The listing builds one solid part. Answer for the finished solid, in the listing's coordinates (mm). A direction names the side the tool comes from. Give positions to 0.01 mm unless a question says otherwise; leave off trailing zeros. Loops run counter-clockwise (first coordinate to the right, second up) from the corner with the lowest first, then second, coordinate; pieces in that order, holes last. Notation, with made-up numbers: M 86,75.25 L 102,75.25 A16 cw 102,105.25 Z; hole C -35,29.5 d4. An arc over 180 degrees is marked long. Return JSON: item names as keys, results as strings.
from build123d import *

# Parameters (mm, degrees)
BOSS_EXTRUDE1_DEPTH = 2.4765


with BuildPart() as part:
    # Sketch1 → Boss-Extrude1 (new, symmetric)
    with BuildSketch(Plane(origin=(0, 0, 0), x_dir=(1, 0, 0), z_dir=(0, 1, 0))):
        with BuildLine():
            Line((-49.53, 45.72), (49.53, 45.72))
            Line((49.53, 45.72), (49.53, 38.1))
            Line((49.53, 38.1), (55.626, 38.1))
            Line((55.626, 38.1), (55.626, 27.94))
            Line((55.626, 27.94), (49.53, 27.94))
            Line((49.53, 27.94), (49.53, 1.208143374))
            Line((49.53, 1.208143374), (55.626, 1.208143374))
            Line((55.626, 1.208143374), (55.626, -8.951856626))
            Line((55.626, -8.951856626), (49.53, -8.951856626))
            Line((49.53, -8.951856626), (49.53, -16.571856626))
            Line((49.53, -16.571856626), (55.626, -16.571856626))
            Line((55.626, -16.571856626), (55.626, -29.271856626))
            Line((55.626, -29.271856626), (21.019827136, -42.136821893))
            ThreePointArc((21.019827136, -42.136821893), (17.95098831, -44.911778638), (17.631953735, -49.036869377))
            Line((17.631953735, -49.036869377), (25.187729856, -73.287029113))
            ThreePointArc((25.187729856, -73.287029113), (26.234780075, -75.207903536), (27.939063878, -76.579577488))
            ThreePointArc((27.939063878, -76.579577488), (41.468907088, -82.632484358), (55.626, -87.022365809))
            Line((55.626, -87.022365809), (55.626, -132.617292876))
            Line((55.626, -132.617292876), (-49.53, -132.617292876))
            Line((-49.53, -132.617292876), (-49.53, -124.997292876))
            Line((-49.53, -124.997292876), (-55.626, -124.997292876))
            Line((-55.626, -124.997292876), (-55.626, -116.107292876))
            Line((-55.626, -116.107292876), (-49.53, -116.107292876))
            Line((-49.53, -116.107292876), (-49.53, -105.947292876))
            Line((-49.53, -105.947292876), (-55.626, -105.947292876))
            Line((-55.626, -105.947292876), (-55.626, -97.057292876))
            Line((-55.626, -97.057292876), (-49.53, -97.057292876))
            Line((-49.53, -97.057292876), (-49.53, -85.359826344))
            ThreePointArc((-49.53, -85.359826344), (-38.527111219, -81.479756652), (-27.939063878, -76.579577488))
            ThreePointArc((-27.939063878, -76.579577488), (-26.234780075, -75.207903536), (-25.187729856, -73.287029113))
            Line((-25.187729856, -73.287029113), (-17.631953735, -49.036869377))
            ThreePointArc((-17.631953735, -49.036869377), (-17.95098831, -44.911778638), (-21.019827136, -42.136821893))
            Line((-21.019827136, -42.136821893), (-55.626, -29.271856626))
            Line((-55.626, -29.271856626), (-55.626, -16.571856626))
            Line((-55.626, -16.571856626), (-49.53, -16.571856626))
            Line((-49.53, -16.571856626), (-49.53, -8.951856626))
            Line((-49.53, -8.951856626), (-55.626, -8.951856626))
            Line((-55.626, -8.951856626), (-55.626, 1.208143374))
            Line((-55.626, 1.208143374), (-49.53, 1.208143374))
            Line((-49.53, 1.208143374), (-49.53, 27.94))
            Line((-49.53, 27.94), (-55.626, 27.94))
            Line((-55.626, 27.94), (-55.626, 38.1))
            Line((-55.626, 38.1), (-49.53, 38.1))
            Line((-49.53, 38.1), (-49.53, 45.72))
        make_face()
    extrude(amount=BOSS_EXTRUDE1_DEPTH, both=True)


solid = part.part
(1) Determine the mould class of faces 1 (the flat face through (-53, 0, 97.057)), 2 (the flat face through (1, -2.476, 42)), 3 (the flat face through (1, 2.476, 42)) for opening direction Y: released by +Y, released by -Y, zero draft, split by the parting line, or undercut.
Values follow:
{"face 1": "zero draft", "face 2": "released by -Y", "face 3": "released by +Y"}
(2) The part is cut by section A-A (x = 41.5). Determine the outline of the cut face in (y, z), and give its area (3 significant figures).
Values follow:
{"outline": "M -2.48,-45.72 L 2.48,-45.72 L 2.48,34.52 L -2.48,34.52 Z; M -2.48,82.64 L 2.48,82.64 L 2.48,132.62 L -2.48,132.62 Z", "area": "645 mm²"}
(3) Given pin 1 (2 mm diameter, centred on y = 1, z = 67, fed in from +X); pin 2 (2.5 mm diameter, centred on y = 0.5, z = 12.5, fed in from +X); pin 3 (2.5 mm diameter, centred on x = -51.5, y = 0, fed in from -Z), each flat-ended and moving along its own axis, determine where each tip first touches the part or whether it passes through.
Values follow:
{"pin 1": "x = 23.54", "pin 2": "x = 49.53", "pin 3": "z = -38.1"}
(4) A tool of negligible diameter and unlimited length cuts with its end or side. For faces 4 (the flat face through (-53, 0, 124.997)), 5 (the flat face through (-53, 0, 116.107)), 6 (the flat face through (49.53, 0, 13)), from which of +Z, -Z, +X, -X, +Y, -Y can it reach the whole face along a straight path? Write none if from no direction.
Values follow:
{"face 4": "+Z, -X, +Y, -Y", "face 5": "-X, +Y, -Y", "face 6": "+X, +Y, -Y"}
(5) The part is cut by section D-D (z = 65.5). Determine the outline of the cut face in (x, y), and give its area (3 significant figures).
Values follow:
{"outline": "M -22.76,-2.48 L 22.76,-2.48 L 22.76,2.48 L -22.76,2.48 Z", "area": "225 mm²"}
(6) The part is cut by section B-B (x = -35.5). Determine the outline of the cut face in (y, z), and give its area (3 significant figures).
Values follow:
{"outline": "M -2.48,-45.72 L 2.48,-45.72 L 2.48,36.75 L -2.48,36.75 Z; M -2.48,80.2 L 2.48,80.2 L 2.48,132.62 L -2.48,132.62 Z", "area": "668 mm²"}
(7) Straight lines are drawn through the part: line 1 along Z through (x, y) = (51.5, 0.15); line 2 along Z through (x, y) = (-50, -0.65); line 3 along X through (y, z) = (2.15, 88). For each, find the intervals that lie inside material, in ascending order.
Values follow:
{"line 1": "-38.1 to -27.94, -1.21 to 8.95, 16.57 to 30.81, 85.93 to 132.62", "line 2": "-38.1 to -27.94, -1.21 to 8.95, 16.57 to 31.36, 97.06 to 105.95, 116.11 to 125", "line 3": "-49.53 to 55.63"}
(8) The part is cut by section C-C (z = -3). Determine the outline of the cut face in (x, y), and give its area (3 significant figures).
Values follow:
{"outline": "M -49.53,-2.48 L 49.53,-2.48 L 49.53,2.48 L -49.53,2.48 Z", "area": "491 mm²"}
